```python
from build123d import *

# Parameters (mm, degrees)
EXTRUDE1_DEPTH  = 60
SKETCH6_R       = 0.5
EXTRUDE2_DEPTH  = 61
LPATTERN1_COUNT = 3
LPATTERN1_PITCH = 15


with BuildPart() as part:
    # Sketch1 → Extrude1 (new body)
    with BuildSketch(Plane(origin=(0, 0, 0), x_dir=(0, 0, -1), z_dir=(1, 0, 0))):
        with BuildLine():
            Line((-3.5, 0.5), (-3, 0))
            Line((-3, 0), (3, 0))
            Line((3, 0), (3.5, 0.5))
            Line((3.5, 0.5), (3.5, 2.465153077))
            ThreePointArc((3.5, 2.465153077), (3.211148341, 2.591798371), (2.999904622, 2.826))
            Line((2.999904622, 2.826), (2.572, 2.90145113))
            ThreePointArc((2.572, 2.90145113), (2.501845147, 2.968757157), (2.45, 3.051))
            Line((2.45, 3.051), (2.45, 3.349))
            ThreePointArc((2.45, 3.349), (2.501845147, 3.431242843), (2.572, 3.49854887))
            Line((2.572, 3.49854887), (2.999904622, 3.574))
            ThreePointArc((2.999904622, 3.574), (3.211148341, 3.808201629), (3.5, 3.934846923))
            Line((3.5, 3.934846923), (3.5, 4.6))
            ThreePointArc((3.5, 4.6), (3.382052634, 4.824039475), (3.2, 5))
            Line((3.2, 5), (-3.2, 5))
            ThreePointArc((-3.2, 5), (-3.382052634, 4.824039475), (-3.5, 4.6))
            Line((-3.5, 4.6), (-3.5, 3.934846923))
            ThreePointArc((-3.5, 3.934846923), (-3.211148341, 3.808201629), (-2.999904622, 3.574))
            Line((-2.999904622, 3.574), (-2.572, 3.49854887))
            ThreePointArc((-2.572, 3.49854887), (-2.501845147, 3.431242843), (-2.45, 3.349))
            Line((-2.45, 3.349), (-2.45, 3.051))
            ThreePointArc((-2.45, 3.051), (-2.501845147, 2.968757157), (-2.572, 2.90145113))
            Line((-2.572, 2.90145113), (-2.999904622, 2.826))
            ThreePointArc((-2.999904622, 2.826), (-3.211148341, 2.591798371), (-3.5, 2.465153077))
            Line((-3.5, 2.465153077), (-3.5, 0.5))
        make_face()
    extrude(amount=EXTRUDE1_DEPTH)

    # Sketch2 → Cut-Revolve1 (revolve, cut)
    with BuildSketch(Plane(origin=(0, 0, 0), x_dir=(-1, 0, 0), z_dir=(0, 0, -1))):
        Polygon((-7.5, 5), (-5.4, 5), (-5.4, 2.7), (-6.3, 2.7), (-6.3, 0.2), (-6.1, 0), (-7.5, 0), align=None)
    revolve(axis=Axis((7.5, 0, 0), (0, 1, 0)), mode=Mode.SUBTRACT)

    # Sketch3 → Cut-Revolve2 (revolve, cut)
    with BuildSketch(Plane(origin=(45, 0, 0), x_dir=(-1, 0, 0), z_dir=(0, 0, -1))):
        Polygon((-7.5, 5), (-5.4, 5), (-5.4, 2.7), (-6.3, 2.7), (-6.3, 0.2), (-6.1, 0), (-7.5, 0), align=None)
    cut_revolve2 = revolve(axis=Axis((52.5, 0, 0), (0, 1, 0)), mode=Mode.SUBTRACT)

    # Sketch6 → Extrude2 (cut, through all)
    with BuildSketch(Plane(origin=(0, 0, 0), x_dir=(0, 0, -1), z_dir=(1, 0, 0))):
        with Locations((1.5, -0.3)):
            Circle(SKETCH6_R)
    extrude(amount=EXTRUDE2_DEPTH, mode=Mode.SUBTRACT)

    # LPattern1: Cut-Revolve2 ×3
    with Locations(*[(-i * LPATTERN1_PITCH, 0, 0) for i in range(1, LPATTERN1_COUNT)]):
        add(cut_revolve2, mode=Mode.SUBTRACT)


solid = part.part
```
Could you check a few things on this model? Use its own coordinates, in mm. A direction names the side the tool comes from. Coordinates: 2 decimals unless noted, no trailing zeros. Loops run counter-clockwise (first coordinate to the right, second up) from the corner with the lowest first, then second, coordinate; pieces in that order, holes last. Notation, with made-up numbers: M 58,-0.5 L 112,-0.5 A21 ccw 112,31.5 Z; hole C 71,-1 d3. An arc over 180 degrees is marked long. Put each result on its own line as item: value. Start each with the question number.
(1) Thinking about a two-plate mould opening in Z: for faces 3 (the face through (30, 1, 3.5)), 4 (the face through (51.355, 1.432, 0.36)), 5 (the face through (60, 3, 0)), 6 (the face through (6, 2.7, 0)), which applies, pulls with the +Z half, pulls with the -Z half, needs draft (parallel to the pull), parting line crosses it, or undercut?
(2) I need wall thicknesses on line 1 (Z direction, x = 22.5, y = 3.8); line 2 (X direction, y = 2.05, z = 1); line 3 (Z direction, x = 37.5, y = 4.35). Which ranges of each line are inside material? Lowest first, please. Write a range as from..to.
(3) Suppose I cut it at A-A on x = 33.5. Please give me the cut outline in (y, z).
(4) Will these pins go through, and if not, where does the flat tip stop? P1, Ø1.9, axis at x = 52.5, z = 0, coming from the +Y side; P2, Ø2, axis at x = 7, z = 0, coming from the +Y side; P3, Ø2.5, axis at x = 52.5, z = 0, coming from the -Y side.
(5) For faces 1 (the face through (20.56, 3.83, -0.8)), 2 (the face through (30, 0, 1)), which set-ups out of +Z, -Z, +X, -X, +Y, -Y let a thin tool reach every point of the face, with its end or its side?
(6) Suppose I cut it at C-C on z = 0. Count the separate pieces of the cut face and the enclosed holes in it, then the cut area to 3 significant figures.
(7) Suppose I cut it at B-B on y = 1.95. Please give me the cut outline in (x, z).
Solutions:
1. face 3: pulls with the +Z half
1. face 4: undercut
1. face 5: needs draft
1. face 6: undercut
2. line 1: z = -3.2..-2.1, 2.1..3.2
2. line 2: x = 0..6.84, 8.16..21.84, 23.16..36.84, 38.16..51.84, 53.16..60
2. line 3: z = -3.5..-2.1, 2.1..3.5
3. outline: M 0,-3 L 0.5,-3.5 L 2.47,-3.5 A0.75 cw 2.83,-3 L 2.9,-2.57 A0.4 cw 3.05,-2.45 L 3.35,-2.45 A0.4 cw 3.5,-2.57 L 3.57,-3 A0.75 cw 3.93,-3.5 L 4.6,-3.5 A0.8 ccw 5,-3.2 L 5,3.2 A0.8 ccw 4.6,3.5 L 3.93,3.5 A0.75 cw 3.57,3 L 3.5,2.57 A0.4 cw 3.35,2.45 L 3.05,2.45 A0.4 cw 2.9,2.57 L 2.83,3 A0.75 cw 2.47,3.5 L 0.5,3.5 L 0,3 L 0,-1.1 A0.5 cw 0,-1.9 Z
4. P1: passes through
4. P2: stops at y = 2.7
4. P3: stops at y = 0.15
5. face 1: +Y
5. face 2: +Z, -Z, +X, -X, -Y
6. separate pieces: 5
6. enclosed holes: 0
6. area: 235 mm2
7. outline: M 0,-3.5 L 60,-3.5 L 60,3.5 L 0,3.5 Z; hole C 7.5,0 d2.4; hole C 22.5,0 d2.4; hole C 37.5,0 d2.4; hole C 52.5,0 d2.4
